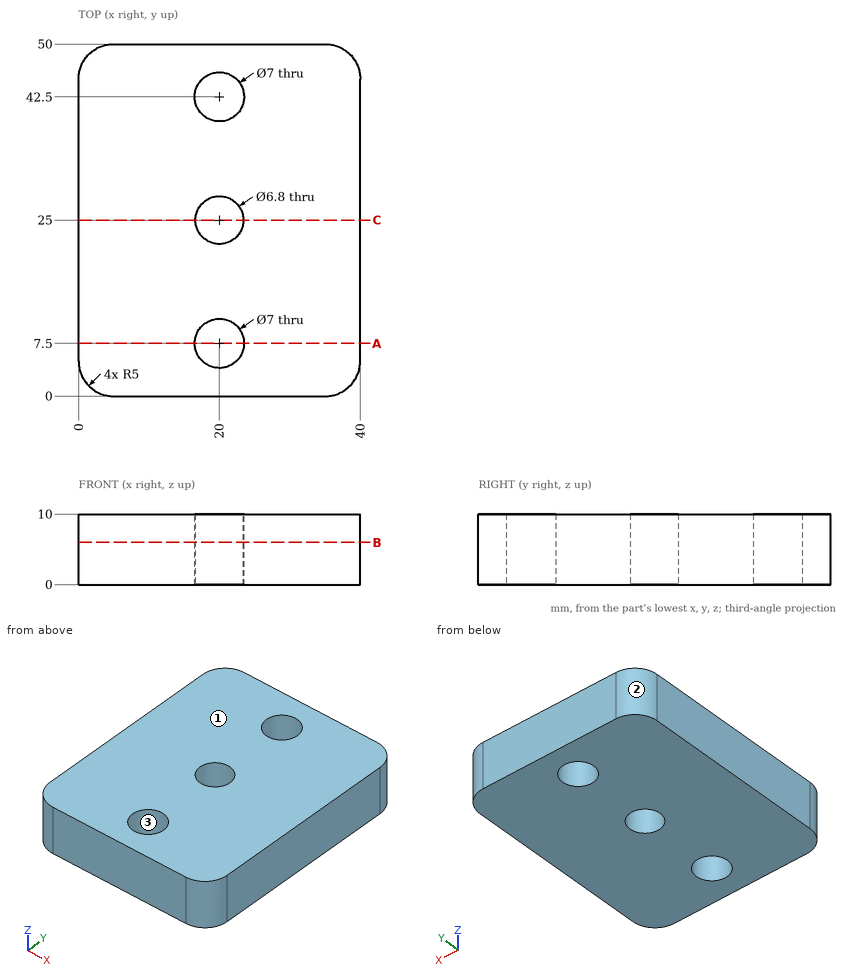
Source: three-view drawing plus pictorial views. Frame: mm from the lowest corner of the part. Give positions to 0.01 mm unless a question says otherwise; leave off trailing zeros. Order: outer loops, then holes, each group sorted by start corner. A loop starts at its lowest first (then second) coordinate and runs counter-clockwise, first axis right, second up. Notation, with made-up numbers: (-0.5, 18.5) -> (57.5, 18.5) arc R16 cw to (57.5, 43.5) -> close; hole circle Ø5 at (30, -3.5). An arc over 180 degrees is marked (long way). Put each result on its own line as item: value.
Q1. Section A-A, the plane y = 7.5. Return loops of the section in (x, z).
Here are the results:
outline: (0, 0) -> (16.5, 0) -> (16.5, 10) -> (0, 10) -> close; (23.5, 0) -> (40, 0) -> (40, 10) -> (23.5, 10) -> close
Q2. Section B-B, the plane z = 6. Return loops of the section in (x, y).
Here are the results:
outline: (0, 5) arc R5 ccw to (5, 0) -> (35, 0) arc R5 ccw to (40, 5) -> (40, 45) arc R5 ccw to (35, 50) -> (5, 50) arc R5 ccw to (0, 45) -> close; hole circle Ø7 at (20, 7.5); hole circle Ø7 at (20, 42.5); hole circle Ø6.8 at (20, 25)
Q3. Section C-C, the plane y = 25. Return loops of the section in (x, z), then the cut area to 3 significant figures.
Here are the results:
outline: (0, 0) -> (16.6, 0) -> (16.6, 10) -> (0, 10) -> close; (23.4, 0) -> (40, 0) -> (40, 10) -> (23.4, 10) -> close
area: 332 mm^2
Q4. Material intervals for L1, parallel to Y at x = 20, z = 6.25; L2, parallel to X at y = 25, z = 2.75; L3, parallel to Y at x = 21, z = 2.5, sorted ascending.
Here are the results:
L1: y = 0 to 4, 11 to 21.6, 28.4 to 39, 46 to 50
L2: x = 0 to 16.6, 23.4 to 40
L3: y = 0 to 4.15, 10.85 to 21.75, 28.25 to 39.15, 45.85 to 50
Q5. Draft query along Y for the marked faces 1, 2 and 3. Return one class per face: released by +Y, released by -Y, zero draft, split by the parting line, or undercut.
Here are the results:
face 1: zero draft
face 2: released by +Y
face 3: undercut
